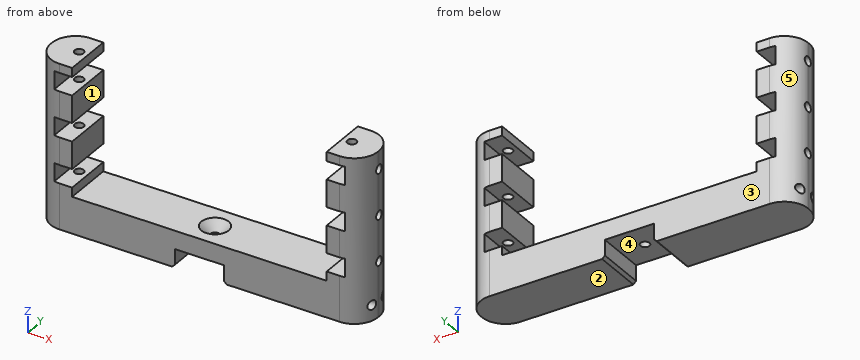
from build123d import *

# Parameters (mm, degrees)
F0_W         = 180
F0_H         = 90
F1_DEPTH     = 27
F2_W         = 140
F2_H         = 70
F3_DEPTH     = 27.001
F4_W         = 10
F4_H         = 10
F5_DEPTH     = 27.001
F6_R         = 2.5
F7_DEPTH     = 80
F9_DEPTH     = 180.001
F10_R        = 2.5
F11_DEPTH    = 20
F12_R        = 2.5
F13_DEPTH    = 20
F14_T1_DEPTH = 155
F15_W        = 27
F15_H        = 10
F16_DEPTH    = 27.0010001
F18_DEPTH    = 90.0010001
F19_SIZE     = 1.5
F20_SIZE     = 5


# Not quite as in the source:
# - a fillet or chamfer that OpenCascade refuses, or shapes differently, is made with other operations: its cross-section is extruded or revolved along the edge and cut away or added


with BuildPart() as f1:
    # F0 (on Front) → F1 (new body)
    with BuildSketch(Plane.XZ):
        with Locations((90, 45)):
            Rectangle(F0_W, F0_H)
    extrude(amount=F1_DEPTH)

    # F2 (on Front) → F3 (cut, through all)
    with BuildSketch(Plane.XZ):
        with Locations((90, 55)):
            Rectangle(F2_W, F2_H)
    extrude(amount=F3_DEPTH, mode=Mode.SUBTRACT)

    # F4 (on Front) → F5 (cut, through all)
    with BuildSketch(Plane.XZ):
        with Locations((165, 80)):
            Rectangle(F4_W, F4_H)
        with Locations((165, 55)):
            Rectangle(F4_W, F4_H)
        with Locations((165, 30)):
            Rectangle(F4_W, F4_H)
        with Locations((15, 30)):
            Rectangle(F4_W, F4_H)
        with Locations((15, 55)):
            Rectangle(F4_W, F4_H)
        with Locations((15, 80)):
            Rectangle(F4_W, F4_H)
    extrude(amount=F5_DEPTH, mode=Mode.SUBTRACT)

    # F6 (on face) → F7 (cut)
    with BuildSketch(Plane.XY.offset(90)):
        with Locations((165, -13)):
            Circle(F6_R)
        with Locations((15, -13)):
            Circle(F6_R)
    extrude(amount=-F7_DEPTH, mode=Mode.SUBTRACT)

    # F8 (on Right) → F9 (cut, through all)
    with BuildSketch(Plane.YZ):
        with BuildLine():
            Line((-13, 77.5), (-13, 82.5))
            ThreePointArc((-13, 82.5), (-15.5, 80), (-13, 77.5))
        make_face()
        with BuildLine():
            ThreePointArc((-13, 77.5), (-11.232233047, 78.232233047), (-10.5, 80))
            ThreePointArc((-10.5, 80), (-11.232233047, 81.767766953), (-13, 82.5))
            Line((-13, 82.5), (-13, 77.5))
        make_face()
        with BuildLine():
            Line((-13, 52.5), (-13, 57.5))
            ThreePointArc((-13, 57.5), (-15.5, 55), (-13, 52.5))
        make_face()
        with BuildLine():
            ThreePointArc((-10.5, 55), (-11.232233047, 56.767766953), (-13, 57.5))
            Line((-13, 57.5), (-13, 52.5))
            ThreePointArc((-13, 52.5), (-11.232233047, 53.232233047), (-10.5, 55))
        make_face()
        with BuildLine():
            Line((-13, 27.5), (-13, 32.5))
            ThreePointArc((-13, 32.5), (-15.5, 30), (-13, 27.5))
        make_face()
        with BuildLine():
            ThreePointArc((-10.5, 30), (-11.232233047, 31.767766953), (-13, 32.5))
            Line((-13, 32.5), (-13, 27.5))
            ThreePointArc((-13, 27.5), (-11.232233047, 28.232233047), (-10.5, 30))
        make_face()
    extrude(amount=F9_DEPTH, mode=Mode.SUBTRACT)

    # F10 (on Right) → F11 (cut)
    with BuildSketch(Plane.YZ):
        with Locations((-8, 8.5)):
            Circle(F10_R)
        with Locations((-18, 8.5)):
            Circle(F10_R)
    extrude(amount=F11_DEPTH, mode=Mode.SUBTRACT)

    # F12 (on face) → F13 (cut)
    with BuildSketch(Plane.YZ.offset(180)):
        with Locations((-8, 8.5)):
            Circle(F12_R)
        with Locations((-18, 8.5)):
            Circle(F12_R)
    extrude(amount=-F13_DEPTH, mode=Mode.SUBTRACT)

    # F14: fillet of radius 13 on 4 edges, made by hand

    # F14_s2 → F14_t1 (cut)
    with BuildSketch(Plane.XY.offset(-32.5)):
        with BuildLine():
            ThreePointArc((0, -13), (3.8076118446, -3.8076118446), (13, 0))
            Line((13, 0), (0, 0))
            Line((0, 0), (0, -13))
        make_face()
        with BuildLine():
            ThreePointArc((0, -14), (3.8076118446, -23.1923881554), (13, -27))
            Line((13, -27), (0, -27))
            Line((0, -27), (0, -14))
        make_face()
        with BuildLine():
            ThreePointArc((167, -27), (176.1923881554, -23.1923881554), (180, -14))
            Line((180, -14), (180, -27))
            Line((180, -27), (167, -27))
        make_face()
        with BuildLine():
            ThreePointArc((167, 0), (176.1923881554, -3.8076118446), (180, -13))
            Line((180, -13), (180, 0))
            Line((180, 0), (167, 0))
        make_face()
    extrude(amount=F14_T1_DEPTH, mode=Mode.SUBTRACT)

    # F15 (on face) → F16 (cut, through all)
    with BuildSketch(Plane.XZ.offset(27)):
        with Locations((90, 5)):
            Rectangle(F15_W, F15_H)
    extrude(amount=-F16_DEPTH, mode=Mode.SUBTRACT)

    # F17 (on Top) → F18 (cut, through all)
    with BuildSketch(Plane.XY):
        with BuildLine():
            Line((87.5, -13.5), (92.5, -13.5))
            ThreePointArc((92.5, -13.5), (90, -11), (87.5, -13.5))
        make_face()
        with BuildLine():
            ThreePointArc((87.5, -13.5), (90, -16), (92.5, -13.5))
            Line((92.5, -13.5), (87.5, -13.5))
        make_face()
    extrude(amount=F18_DEPTH, mode=Mode.SUBTRACT)

    # F19
    f19_edges = [f1.edges().sort_by_distance(p)[0] for p in [
        (76.5, -13.5, 0),
        (103.5, -13.5, 0),
    ]]
    chamfer(f19_edges, length=F19_SIZE)

    # F20
    f20_edges = [f1.edges().sort_by_distance(p)[0] for p in [
        (92.5, -13.5, 20),
    ]]
    chamfer(f20_edges, length=F20_SIZE)


solid = f1.part
Work out the finished part from the listing and answer in its coordinate system (mm). Face numbers are marked on the shaded views. A direction names the side the tool comes from. Round coordinates to 2 decimals unless told otherwise and drop trailing zeros. Write each loop counter-clockwise with the first axis right and the second up, starting at its lowest first coordinate (ties: lowest second). Pieces come first, ordered by that corner, then holes. Notation, with made-up numbers: (12.5, -34) - (58.5, -34) arc R18 cw to (58.5, -13) - close; hole circle Ø2 at (-36.5, -31.5). An arc over 180 degrees is marked (long way). Answer in a Markdown table with one row per item. Add a question column.
1. The mould has two halves that part along X. Classify the marked faces 3, 4 and 5: +X half, -X half, draft (parallel to the pull), parting line (faces both ways), or undercut.
2. Given pin 1 (3 mm diameter, centred on y = -10, z = 28, fed in from -X); pin 2 (4.5 mm diameter, centred on y = -18, z = 8.5, fed in from +X); pin 3 (1.5 mm diameter, centred on y = -18.5, z = 31.5, fed in from +X), each flat-ended and moving along its own axis, determine where each tip first touches the part or whether it passes through.
3. For the marked faces 1 and 2, determine the directions among +Z, -Z, +X, -X, +Y, -Y from which every point of the face is accessible in a straight line to the end or side of a thin tool.
4. Find the intervals of material crossed by line 1 along Z through (x, y) = (167.5, -8); line 2 along Y through (x, z) = (14, 8.5); line 3 along Z through (x, y) = (173.75, -8), in increasing order. Write a range as from..to.
5. A cutting plane is placed at A-A, the plane x = 165. Count the separate pieces of the cut face and the enclosed holes in it, and give its area (3 significant figures).
6. A cutting plane is placed at B-B, the plane x = 35.5. Determine the outline of the cut face in (y, z).
Worked out:
| question | item | result |
|---|---|---|
| 1 | face 3 | draft |
| 1 | face 4 | undercut |
| 1 | face 5 | -X half |
| 2 | pin 1 | x = 0.09 |
| 2 | pin 2 | x = 160 |
| 2 | pin 3 | x = 179.45 |
| 3 | face 1 | +Z, +Y, -Y |
| 3 | face 2 | -Z, +X, -X, +Y, -Y |
| 4 | line 1 | 0..6, 11..25, 35..50, 60..75, 85..90 |
| 4 | line 2 | -27..-20.5, -15.5..-10.5, -5.5..0 |
| 4 | line 3 | 0..6, 11..90 |
| 5 | separate pieces | 7 |
| 5 | enclosed holes | 2 |
| 5 | area | 1,330 mm^2 |
| 6 | outline | (-27, 0) - (0, 0) - (0, 20) - (-27, 20) - close |
